from build123d import *

# Parameters (mm, degrees)
SKETCH_1_R          = 11
EXTRUDE_1_DEPTH     = 2
SKETCH_2_R          = 9
EXTRUDE_2_DEPTH     = 2.4
SKETCH_3_R          = 10
CUT_EXTRUDE_1_DEPTH = 1
SKETCH_4_R          = 8
CUT_EXTRUDE_2_DEPTH = 10
CUT_EXTRUDE_3_DEPTH = 2


with BuildPart() as part:
    # 草图1 → 凸台-拉伸1 (new body)
    with BuildSketch(Plane.XY):
        Circle(SKETCH_1_R)
    extrude(amount=EXTRUDE_1_DEPTH)

    # 草图2 → 凸台-拉伸2 (add)
    with BuildSketch(Plane.XY.offset(2)):
        Circle(SKETCH_2_R)
    extrude(amount=EXTRUDE_2_DEPTH)

    # 草图3 → 切除-拉伸1 (cut)
    with BuildSketch(Plane(origin=(0, 0, 0), x_dir=(-1, 0, 0), z_dir=(0, 0, -1))):
        Circle(SKETCH_3_R)
    extrude(amount=-CUT_EXTRUDE_1_DEPTH, mode=Mode.SUBTRACT)

    # 草图4 → 切除-拉伸2 (cut)
    with BuildSketch(Plane(origin=(0, 0, 1), x_dir=(-1, 0, 0), z_dir=(0, 0, -1))):
        Circle(SKETCH_4_R)
    extrude(amount=-CUT_EXTRUDE_2_DEPTH, mode=Mode.SUBTRACT)

    # 草图5 → 切除-拉伸3 (cut)
    with BuildSketch(Plane.XY.offset(4.4)):
        with BuildLine():
            Line((0, 0), (6.363961031, 6.363961031))
            ThreePointArc((6.363961031, 6.363961031), (9, 0), (6.363961031, -6.363961031))
            Line((6.363961031, -6.363961031), (0, 0))
        make_face()
    extrude(amount=-CUT_EXTRUDE_3_DEPTH, mode=Mode.SUBTRACT)


solid = part.part
Geometry check sheet. Reference: the model listing, model coordinates, mm. A direction names the side the tool comes from. Coordinates: 2 decimals unless noted, no trailing zeros. Write each loop counter-clockwise with the first axis right and the second up, starting at its lowest first coordinate (ties: lowest second). Pieces come first, ordered by that corner, then holes. Notation, with made-up numbers: (33.5, -13.5) -> (43.5, -13.5) arc R20 cw to (43.5, 15.5) -> close; hole circle Ø4 at (20, -10). An arc over 180 degrees is marked (long way). One line per question, with ' | ' between items.
1. Cross-section at B-B on x = 0. Record the cut outline in (y, z), and give its area (3 significant figures).
Answers:
outline: (-11, 0) -> (-10, 0) -> (-10, 1) -> (-8, 1) -> (-8, 4.4) -> (-9, 4.4) -> (-9, 2) -> (-11, 2) -> close; (8, 1) -> (10, 1) -> (10, 0) -> (11, 0) -> (11, 2) -> (9, 2) -> (9, 4.4) -> (8, 4.4) -> close | area: 12.8 mm²
2. Cross-section at A-A on y = 0. Record the cut outline in (x, z), and give its area (3 significant figures).
Answers:
outline: (-11, 0) -> (-10, 0) -> (-10, 1) -> (-8, 1) -> (-8, 4.4) -> (-9, 4.4) -> (-9, 2) -> (-11, 2) -> close; (8, 1) -> (10, 1) -> (10, 0) -> (11, 0) -> (11, 2) -> (9, 2) -> (9, 2.4) -> (8, 2.4) -> close | area: 10.8 mm²
3. Depth check by flat-ended pin: pin 1 Ø8 at (x, y) = (-5, 1) entering from -Z; pin 2 Ø2 at (y, z) = (-5, 1) entering from -X; pin 3 Ø6 at (x, y) = (3.5, 1.5) entering from -Z; pin 4 Ø3.5 at (x, y) = (7.5, -1.5) entering from +Z. Enter the tip coordinate at first touch or a pass-through.
Answers:
pin 1: stops at z = 1 | pin 2: stops at x = -10.25 | pin 3: passes through | pin 4: stops at z = 2.4
4. Set-up check for faces 4 (the flat face through (0, 8.2, 1)), 5 (the cylindrical face through (-2.38, -10.74, 0.99)), 6 (the flat face through (2, -9, 2)): record each of +Z, -Z, +X, -X, +Y, -Y from which the full face is reachable in a straight line by a thin tool's end or side.
Answers:
face 4: -Z | face 5: +Z, -Z | face 6: +Z
5. Thickness scan on probe 1 along Y at (x, z) = (0, 0.7); probe 2 along X at (y, z) = (5.75, 0.4); probe 3 along Y at (x, z) = (0, 3.7). Record the ranges inside material, lowest first. Write a range as from..to.
Answers:
probe 1: y = -11..-10, 10..11 | probe 2: x = -9.38..-8.18, 8.18..9.38 | probe 3: y = -9..-8, 8..9
6. Cross-section at C-C on z = 3.7. Record the cut outline in (x, y), and give its area (3 significant figures).
Answers:
outline: (5.66, -5.66) arc R8 cw (long way) to (5.66, 5.66) -> (6.36, 6.36) arc R9 ccw (long way) to (6.36, -6.36) -> close | area: 40.1 mm²
7. Draft check along Y on faces 1 (the cylindrical face through (-9, 0, 3)), 2 (the cylindrical face through (2.17, -9.76, 0.49)), 3 (the flat face through (-8, -3, 4.4)). Enter one of: +Y half, -Y half, draft (parallel to the pull), parting line (faces both ways), or undercut.
Answers:
face 1: parting line | face 2: undercut | face 3: draft
